CAD build for the part. Positions are in the model's coordinates, mm. Give positions to 0.01 mm unless a question says otherwise; leave off trailing zeros. Answer as CSV lines item,"result".
```python
from build123d import *

# Parameters (mm, degrees)
SKETCH_1_W      = 50
SKETCH_1_H      = 70
SKETCH_1_R      = 1.5
EXTRUDE_1_DEPTH = 2
FILLET_1_R      = 3


with BuildPart() as part:
    # 草图1 → 凸台-拉伸1 (new body)
    with BuildSketch(Plane(origin=(0, 0, 0), x_dir=(1, 0, 0), z_dir=(0, 1, 0))):
        Rectangle(SKETCH_1_W, SKETCH_1_H)
        with Locations(Location((20.505712162, 32.246478585, 0), (0, 0, 270))):
            Circle(SKETCH_1_R, mode=Mode.SUBTRACT)
        with Locations(Location((-20.505712162, 32.246478585, 0), (0, 0, 90))):
            Circle(SKETCH_1_R, mode=Mode.SUBTRACT)
        with Locations(Location((21.261079234, -31.753521415, 0), (0, 0, 90))):
            Circle(SKETCH_1_R, mode=Mode.SUBTRACT)
        with Locations(Location((-19.738920766, -32.721470313, 0), (0, 0, 270))):
            Circle(SKETCH_1_R, mode=Mode.SUBTRACT)
    extrude(amount=EXTRUDE_1_DEPTH)

    # 圆角1
    fillet_1_edges = [part.edges().sort_by_distance(p)[0] for p in [
        (25, 1, 35),
        (-25, 1, 35),
        (-25, 1, -35),
        (25, 1, -35),
    ]]
    fillet(fillet_1_edges, radius=FILLET_1_R)


solid = part.part
```
1) Pin check, flat tip, straight feed: P1, Ø12, axis at x = 12.5, z = -0.5, coming from the -Y side. Stop position of the tip, or through.
Data:
P1,"stops at y = 0"
2) Pull direction X, two halves, no side cores. Call faces 1 (the cylindrical face through (24.1, 1.01, 34.14)), 2 (the cylindrical face through (-18.725, 0.986, 31.616)), 3 (the flat face through (0, 0, 0)): pulls with the +X half, pulls with the -X half, needs draft (parallel to the pull), parting line crosses it, or undercut.
Data:
face 1,"pulls with the +X half"
face 2,"undercut"
face 3,"needs draft"
3) Wall check: line 1 along X through (y, z) = (0.8, -31); line 2 along Z through (x, y) = (-20.5, 0.2); line 3 along X through (y, z) = (0.4, 32). Give the ranges that are in metal, low to high. Write a range as [from, to].
Data:
line 1,"x = [-25, -21.34], [-19.67, 19.67], [21.34, 25]"
line 2,"z = [-35, -33.75], [-30.75, 31.43], [34.01, 35]"
line 3,"x = [-25, -21.05], [-18.42, 19.78], [22.74, 25]"
